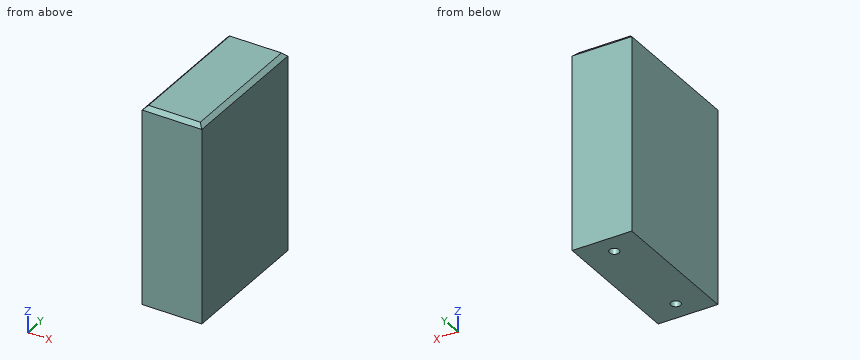
from build123d import *

# Parameters (mm, degrees)
F0_W     = 30
F0_H     = 100
F1_DEPTH = 70
F2_R     = 2.446969
F3_DEPTH = 15
F4_SIZE  = 2


with BuildPart() as f1:
    # F0 (on Front) → F1 (new body)
    with BuildSketch(Plane.XZ):
        with Locations((4.792286, 3.770108)):
            Rectangle(F0_W, F0_H)
    extrude(amount=F1_DEPTH)

    # F2 (on face) → F3 (cut)
    with BuildSketch(Plane(origin=(0, 0, -46.229892), x_dir=(1, 0, 0), z_dir=(0, 0, -1))):
        with Locations((4.792286, 60)):
            Circle(F2_R)
        with Locations((4.792286, 10)):
            Circle(F2_R)
    extrude(amount=-F3_DEPTH, mode=Mode.SUBTRACT)

    # F4
    f4_edges = [f1.edges().sort_by_distance(p)[0] for p in [
        (4.792286, -70, 53.770108),
        (19.792286, -35, 53.770108),
        (4.792286, 0, 53.770108),
        (-10.207714, -35, 53.770108),
    ]]
    chamfer(f4_edges, length=F4_SIZE)


solid = f1.part
Design review of the part built by this model. Coordinates are the model's own, in mm. Give positions to 0.01 mm unless a question says otherwise; leave off trailing zeros. Write each loop counter-clockwise with the first axis right and the second up, starting at its lowest first coordinate (ties: lowest second). Pieces come first, ordered by that corner, then holes. Notation, with made-up numbers: M 13.5,3 L 52.5,3 A16 ccw 52.5,22 Z; hole C 76.5,34 d7. An arc over 180 degrees is marked long. Answer as a JSON object with one key per item and string values. Group by question number.
1) Clearance check with a flat-ended pin moving along its axis: pin 1 Ø2.5 at (x, y) = (4.5, -10.5) entering from -Z. State where the tip first meets the part, or that it passes through.
2) We need section B-B (x = 5). Give the boundary of the cut face in (y, z).
3) We need section A-A (y = -60). Give the boundary of the cut face in (x, z), and give its area (3 significant figures).
4) For line 1 along X through (y, z) = (-10, -41); line 2 along Y through (x, z) = (5.5, -34), list the stretches that pass through material, from the lowest coordinate up.
Answer key:
{
 "1": {"pin 1": "stops at z = -31.23"},
 "2": {"outline": "M -70,-46.23 L -62.44,-46.23 L -62.44,-31.23 L -57.56,-31.23 L -57.56,-46.23 L -12.44,-46.23 L -12.44,-31.23 L -7.56,-31.23 L -7.56,-46.23 L 0,-46.23 L 0,51.77 L -2,53.77 L -68,53.77 L -70,51.77 Z"},
 "3": {"outline": "M -10.21,-46.23 L 2.35,-46.23 L 2.35,-31.23 L 7.24,-31.23 L 7.24,-46.23 L 19.79,-46.23 L 19.79,51.77 L 17.79,53.77 L -8.21,53.77 L -10.21,51.77 Z", "area": "2,920 mm²"},
 "4": {"line 1": "x = -10.21 to 2.35, 7.24 to 19.79", "line 2": "y = -70 to -62.34, -57.66 to -12.34, -7.66 to 0"}
}
